Can you work these out from the model? Positions are in its coordinate system, mm. A direction names the side the tool comes from. Round coordinates to 2 decimals unless told otherwise and drop trailing zeros. Loops run counter-clockwise (first coordinate to the right, second up) from the corner with the lowest first, then second, coordinate; pieces in that order, holes last. Notation, with made-up numbers: (43, 82) - (95, 82) arc R15 ccw to (95, 106) - close; hole circle Ø5 at (-39.5, 32). An arc over 180 degrees is marked (long way). Answer as CSV lines item,"result".
```python
from build123d import *

# Parameters (mm, degrees)
F1_DEPTH  = 6
F2_R      = 5
F3_W      = 40
F3_H      = 5.699848
F4_DEPTH  = 44
F5_R      = 5
F7_DEPTH  = 25
F8_W      = 6
F8_H      = 6
F9_DEPTH  = 36.3
F10_R     = 3
F11_DEPTH = 25
F13_DEPTH = 49.1


with BuildPart() as f1:
    # F0 (on Top) → F1 (new body)
    with BuildSketch(Plane.XY):
        Polygon((-30.455219, 30), (-30.455219, 0), (-30.455219, -10), (9.544781, -10), (9.544781, 30), align=None)
    extrude(amount=F1_DEPTH)

    # F2
    f2_edges = [f1.edges().sort_by_distance(p)[0] for p in [
        (-30.455219, -10, 3),
        (9.544781, -10, 3),
    ]]
    fillet(f2_edges, radius=F2_R)

    # F3 (on face) → F4 (join)
    with BuildSketch(Plane.XY.offset(6)):
        with Locations((-10.455219, 27.150076)):
            Rectangle(F3_W, F3_H)
    extrude(amount=F4_DEPTH)

    # F5
    f5_edges = [f1.edges().sort_by_distance(p)[0] for p in [
        (-30.455219, 27.150076, 50),
        (9.544781, 27.150076, 50),
    ]]
    fillet(f5_edges, radius=F5_R)

    # F6 (on face) → F7 (cut)
    with BuildSketch(Plane.XZ.offset(-24.300152)):
        Polygon((-21.955219, 8.545761), (-25.455219, 45), (-25.455219, 8.545761), align=None)
        Polygon((-20.455219, 45), (-22.955219, 45), (-19.455219, 8.545761), (-16.955219, 8.545761), align=None)
        Polygon((-15.455219, 45), (-17.955219, 45), (-14.455219, 8.545761), (-11.955219, 8.545761), align=None)
        Polygon((-5.455219, 45), (-8.955219, 8.545761), (-6.455219, 8.545761), (-2.955219, 45), align=None)
        Polygon((-0.455219, 45), (-3.955219, 8.545761), (-1.455219, 8.545761), (2.044781, 45), align=None)
        Polygon((4.544781, 45), (1.044781, 8.545761), (4.544781, 8.545761), align=None)
    extrude(amount=-F7_DEPTH, mode=Mode.SUBTRACT)

    # F8 (on face) → F9 (join)
    with BuildSketch(Plane(origin=(0, 0, 0), x_dir=(1, 0, 0), z_dir=(0, 0, -1))):
        with BuildLine():
            Line((-30.455219, 5), (-30.455219, 4))
            Line((-30.455219, 4), (-24.455219, 4))
            Line((-24.455219, 4), (-24.455219, 10))
            Line((-24.455219, 10), (-25.455219, 10))
            ThreePointArc((-25.455219, 10), (-28.990753, 8.535534), (-30.455219, 5))
        make_face()
        with BuildLine():
            Line((4.544781, 10), (3.544781, 10))
            Line((3.544781, 10), (3.544781, 4))
            Line((3.544781, 4), (9.544781, 4))
            Line((9.544781, 4), (9.544781, 5))
            ThreePointArc((9.544781, 5), (8.080315, 8.535534), (4.544781, 10))
        make_face()
        with Locations((-27.455219, -27)):
            Rectangle(F8_W, F8_H)
        with Locations((6.544781, -27)):
            Rectangle(F8_W, F8_H)
    extrude(amount=F9_DEPTH)

    # F10
    f10_edges = [f1.edges().sort_by_distance(p)[0] for p in [
        (9.544781, 30, 4.35),
    ]]
    fillet(f10_edges, radius=F10_R)

    # F6 (on face) → F11 (cut)
    with BuildSketch(Plane.XZ.offset(-24.300152)):
        Polygon((-7.955219, 45), (-12.955219, 45), (-10.455219, 18.961258), align=None)
    extrude(amount=-F11_DEPTH, mode=Mode.SUBTRACT)

    # F12 (on face) → F13 (cut)
    with BuildSketch(Plane.YZ.offset(9.544781)):
        Polygon((-5, 6), (-5, 5.73364), (24.300152, 4.866716), (24.300152, 6), align=None)
        Polygon((24.300152, 7.596356), (-13.065776, 5.972288), (-5, 5.73364), (-5, 6), (24.300152, 6), align=None)
    extrude(amount=-F13_DEPTH, mode=Mode.SUBTRACT)


solid = f1.part
```
Q1. I'm going to push flat-ended pins straight in: pin 1 Ø3 at (x, z) = (1, 27) entering from -Y; pin 2 Ø3 at (x, y) = (0.5, 26.5) entering from -Z; pin 3 Ø3 at (y, z) = (28, -26) entering from +X; pin 4 Ø6 at (x, y) = (-18, 10) entering from +Z. Where does each tip first touch, or does it pass through?
Checks:
pin 1,"y = 24.3"
pin 2,"z = 0"
pin 3,"x = 9.54"
pin 4,"z = 5.38"
Q2. We'd pull the mould along X, two halves only. Please class faces 4 (the flat face through (-11.723, 27.11, 32.163)), 5 (the flat face through (7, 24, -18)), 6 (the cylindrical face through (8.69, 29.1, 3.78)): pulls with the +X half, pulls with the -X half, needs draft (parallel to the pull), parting line crosses it, or undercut.
Checks:
face 4,"undercut"
face 5,"needs draft"
face 6,"pulls with the +X half"
Q3. Imagine slicing it at D-D (y = 1). Write out the boundary of the cut face in (x, z).
Checks:
outline,"(-30.46, 0) - (9.54, 0) - (9.54, 5.56) - (-30.46, 5.56) - close"
Q4. Imagine slicing it at B-B (z = 15.5). Count the separate pieces of the cut face and the enclosed holes in it, then the cut area to 3 significant figures.
Checks:
separate pieces,"7"
enclosed holes,"0"
area,"135 mm²"
Q5. Imagine slicing it at A-A (z = -6). Write out the boundary of the cut face in (x, y).
Checks:
outline,"(-30.46, -5) arc R5 ccw to (-25.46, -10) - (-24.46, -10) - (-24.46, -4) - (-30.46, -4) - close; (-30.46, 24) - (-24.46, 24) - (-24.46, 30) - (-27.46, 30) arc R3 ccw to (-30.46, 27) - close; (3.54, -10) - (4.54, -10) arc R5 ccw to (9.54, -5) - (9.54, -4) - (3.54, -4) - close; (3.54, 24) - (9.54, 24) - (9.54, 27) arc R3 ccw to (6.54, 30) - (3.54, 30) - close"
Q6. If I drill on line 1 along X through (y, z) = (27, -30); line 2 along Y through (x, z) = (-26, 36); line 3 along Y through (x, z) = (6, -23.5), over which ranges is the centre line in solid material (lowest first)? Write a range as [from, to].
Checks:
line 1,"[-30.46, -24.46], [3.54, 9.54]"
line 2,"[24.3, 30]"
line 3,"[-9.78, -4], [24, 30]"
Q7. On a 3-axis mill with a long thin cutter (end or side, diameter ignored), from which of +Z, -Z, +X, -X, +Y, -Y can I reach the whole of each face in a straight line? I mean faces 1 (the flat face through (-18.68, 27.11, 26.52)), 2 (the flat face through (-11, 26, 50)), 3 (the flat face through (-27, 24, -18)). Say none if no direction works.
Checks:
face 1,"+Y, -Y"
face 2,"+Z, +X, -X, +Y, -Y"
face 3,"-Z, +X, -X"
Q8. Imagine slicing it at C-C (y = 7.5). Write out the boundary of the cut face in (x, z), then the cut area to 3 significant figures.
Checks:
outline,"(-30.46, 0) - (9.54, 0) - (9.54, 5.36) - (-30.46, 5.36) - close"
area,"215 mm²"
